Could you check a few things on this model? Use its own coordinates, in mm. A direction names the side the tool comes from. Coordinates: 2 decimals unless noted, no trailing zeros. Write each loop counter-clockwise with the first axis right and the second up, starting at its lowest first coordinate (ties: lowest second). Pieces come first, ordered by that corner, then holes. Notation, with made-up numbers: (58.5, 68.5) - (96.5, 68.5) arc R10 ccw to (96.5, 82.5) - close; hole circle Ø7 at (68.5, -2.5). An arc over 180 degrees is marked (long way). Write item = value, one per line. Start each with the question number.
Autodesk Inventor part; units mm, degrees
ref_plane "YZ Plane" through (0, 0, 0) normal (1, 0, 0) x (0, 1, 0)
ref_plane "XZ Plane" through (0, 0, 0) normal (0, 1, 0) x (-1, 0, 0)
ref_plane "XY Plane" through (0, 0, 0) normal (0, 0, 1) x (1, 0, 0)
sketch "Skizze1" plane through (0, 0, 0) normal (0, 0, 1) x (1, 0, 0)
  circle A0 centre (0, 0) radius 8
  circle A1 centre (0, 0) radius 6
  dimension "d0" = 2
  dimension "d1" = 16
extrude "Extrusion1" add sketch "Skizze1" along normal blind 298
sketch "Skizze2" plane through (0, 0, 298) normal (0, 0, 1) x (1, 0, 0)
  circle A0 centre (0, 0) radius 8
  circle A1 centre (0, 0) radius 7
  dimension "d4" = 14
extrude "Extrusion2" cut sketch "Skizze2" against normal blind 50
sketch "Skizze3" plane through (0, 0, 248) normal (0, 0, 1) x (1, 0, 0)
  circle A0 centre (0, 0) radius 8
  circle A1 centre (0, 0) radius 7.75
  dimension "d7" = 15.5
extrude "Extrusion3" cut sketch "Skizze3" against normal through all
sketch "Skizze4" plane through (0, 0, 0) normal (0, 0, -1) x (-1, 0, 0)
  circle A0 centre (0, 0) radius 7.75
  circle A1 centre (0, 0) radius 6
  circle A2 centre (0, 0) radius 8
  dimension "d10" = 16
extrude "Extrusion4" add sketch "Skizze4" against normal blind 9 contours A2
sketch "Skizze5" plane through (0, 0, 0) normal (0, 1, 0) x (-1, 0, 0)
  line L0 (-8, 9) -> (8, 9)
  line L1 (8, 0) -> (-8, 0)
  line L2 (8, 0) -> (8, 9)
  line L3 (6, 0) -> (6, 298)
  line L4 (7.75, 248) -> (7.75, 9)
  line L5 (0, -50) -> (0, 300)
  line L6 (8, 7.5) -> (7.25, 7.5)
  line L7 (7.25, 7.5) -> (7.25, 9)
  line L8 (8, 9) -> (7.25, 9)
  line L9 (8, 9) -> (8, 7.5)
  point P0 (0, 0)
  dimension "d17" = 1.5
  dimension "d18" = 14.5
revolve "Umdrehung1" cut sketch "Skizze5" angle 360 about axis through (0, 0, -10) along (0, 0, 1) contours L0 L2 L6 L7
chamfer "Fase1" distance 0.75 angle 45 1 edges at (8, 0, 7.5)
thread "Gewinde3"
fillet "Rundung1" radius 0.5 1 edges at (-7, 0, 248)
properties part number "13_0204_023"
1) For P1, Ø6, axis at x = -6, z = 171, coming from the -Y side; P2, Ø3, axis at x = -3, z = 129.5, coming from the -Y side; P3, Ø3, axis at y = -0.5, z = 81, coming from the +X side, each with a flat end and sliding along its axis, tell me the tip position at first contact or that it passes through.
2) Suppose I cut it at C-C on z = 36.5. Please give me the cut outline in (x, y).
3) If I drill on probe 1 along Y at (x, z) = (0, 109.5); probe 2 along Z at (x, y) = (-6.25, 4.5); probe 3 along X at (y, z) = (2.25, 269), over which ranges is the centre line in solid material (lowest first)? Write a range as [from, to].
4) Which directions (+Z, -Z, +X, -X, +Y, -Y) give clear straight access to the entire face, cutting with the end or side of a thin tool? Please do faces 1 (the cylindrical face through (6.466, -2.681, 273.596)), 2 (the flat face through (-2.8, 6.9, 9)), 3 (the cylindrical face through (-6, 0, 147)).
5) Thinking about a two-plate mould opening in Z: for faces 4 (the cylindrical face through (1.73, -7.81, 3.33)), 5 (the cylindrical face through (-3.35, 6.43, 8.26)), 6 (the flat face through (6, 2, 298)), which applies, +Z half, -Z half, draft (parallel to the pull), parting line (faces both ways), or undercut?
Reply:
q1.P1 = -7.15
q1.P2 = -7.6
q1.P3 = 7.75
q2.outline = circle Ø15.5 at (0, 0); hole circle Ø12 at (0, 0)
q3.probe_1 = [-7.75, -6], [6, 7.75]
q3.probe_2 = [0, 7.05], [9, 248]
q3.probe_3 = [-6.63, -5.56], [5.56, 6.63]
q4.face_1 = +Z
q4.face_2 = none
q4.face_3 = +Z, -Z
q5.face_4 = draft
q5.face_5 = undercut
q5.face_6 = +Z half
